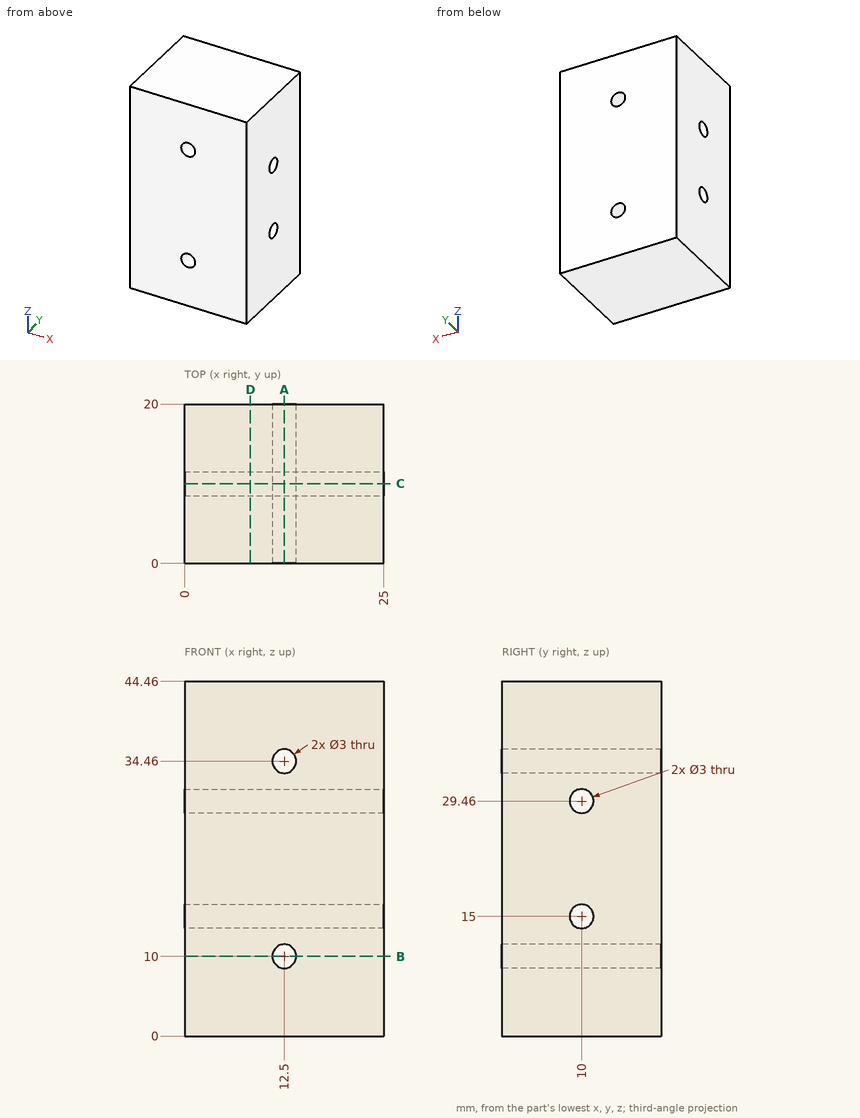
Part print with two shaded views. Sizes in mm from the minimum x, y, z corner. Coordinates: 2 decimals unless noted, no trailing zeros. Loops run counter-clockwise (first coordinate to the right, second up) from the corner with the lowest first, then second, coordinate; pieces in that order, holes last. Notation, with made-up numbers: (-26.75, 60) -> (10.25, 60) arc R18 ccw to (10.25, 90) -> close; hole circle Ø7 at (58, -3.75). An arc over 180 degrees is marked (long way). Answer as a JSON object with one key per item and string values.
Q1. Cut at C-C (y = 10). List the corners of the cut face in (x, z).
Report:
{"outline": "(0, 0) -> (25, 0) -> (25, 13.5) -> (0, 13.5) -> close; (0, 16.5) -> (25, 16.5) -> (25, 27.96) -> (0, 27.96) -> close; (0, 30.96) -> (25, 30.96) -> (25, 44.46) -> (0, 44.46) -> close; hole circle Ø3 at (12.5, 10); hole circle Ø3 at (12.5, 34.46)"}
Q2. Cut at D-D (x = 8.25). List the corners of the cut face in (y, z).
Report:
{"outline": "(0, 0) -> (20, 0) -> (20, 44.46) -> (0, 44.46) -> close; hole circle Ø3 at (10, 15); hole circle Ø3 at (10, 29.46)"}
Q3. Probe probe 1 along Z at (x, y) = (12.5, 5.25); probe 2 along Y at (x, z) = (15.5, 15); probe 3 along Z at (x, y) = (11.5, 4.5). List the from-to ranges inside material, lowest first.
Report:
{"probe 1": "z = 0 to 8.5, 11.5 to 32.96, 35.96 to 44.46", "probe 2": "y = 0 to 8.5, 11.5 to 20", "probe 3": "z = 0 to 8.88, 11.12 to 33.34, 35.58 to 44.46"}
Q4. Cut at B-B (z = 10). List the corners of the cut face in (x, y).
Report:
{"outline": "(0, 0) -> (11, 0) -> (11, 20) -> (0, 20) -> close; (14, 0) -> (25, 0) -> (25, 20) -> (14, 20) -> close"}
Q5. Cut at A-A (x = 12.5). List the corners of the cut face in (y, z).
Report:
{"outline": "(0, 0) -> (20, 0) -> (20, 8.5) -> (0, 8.5) -> close; (0, 11.5) -> (20, 11.5) -> (20, 32.96) -> (0, 32.96) -> close; (0, 35.96) -> (20, 35.96) -> (20, 44.46) -> (0, 44.46) -> close; hole circle Ø3 at (10, 15); hole circle Ø3 at (10, 29.46)"}
